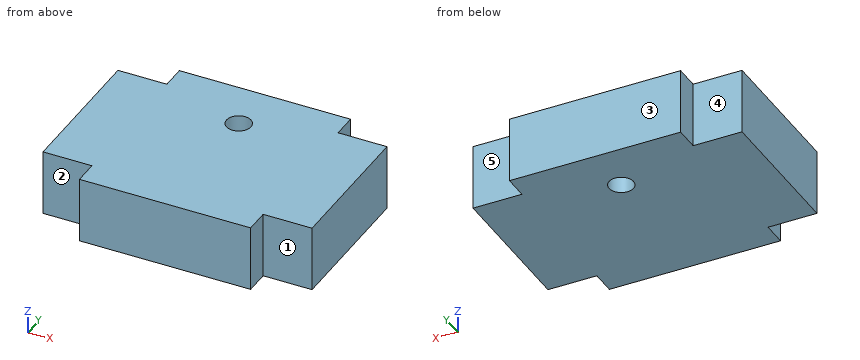
Autodesk Inventor part; units mm, degrees
ref_plane "YZ Plane" through (0, 0, 0) normal (1, 0, 0) x (0, 1, 0)
ref_plane "XZ Plane" through (0, 0, 0) normal (0, 1, 0) x (-1, 0, 0)
ref_plane "XY Plane" through (0, 0, 0) normal (0, 0, 1) x (1, 0, 0)
sketch "Sketch1" plane through (0, 0, 0) normal (0, 0, 1) x (1, 0, 0)
  line L0 (-8.75, -10) -> (8.75, -10)
  line L1 (8.75, -10) -> (8.75, 10)
  line L2 (8.75, 10) -> (-8.75, 10)
  line L3 (-8.75, 10) -> (-8.75, -10)
  line L4 (8.75, 7.5) -> (13.75, 7.5)
  line L5 (13.75, 7.5) -> (13.75, -7.5)
  line L6 (13.75, -7.5) -> (8.75, -7.5)
  line L7 (8.75, -7.5) -> (8.75, 7.5)
  line L8 (-8.75, 7.5) -> (-13.75, 7.5)
  line L9 (-13.75, 7.5) -> (-13.75, -7.5)
  line L10 (-13.75, -7.5) -> (-8.75, -7.5)
  line L11 (-8.75, -7.5) -> (-8.75, 7.5)
  circle A0 centre (0, 4.75) radius 1.25
  point P0 (0, 0)
  point P1 (8.75, 0)
  point P2 (0, 10)
  point P3 (-13.75, 0)
  point P4 (13.75, 0)
  dimension "d0" = 5
  dimension "d1" = 17.5
  dimension "d2" = 20
  dimension "d3" = 15
  dimension "d7" = 8.75
  dimension "d9" = 2.5
  dimension "d10" = 2.5
  dimension "d11" = 4.75
extrude "Extrusion1" add sketch "Sketch1" along normal blind 6.731
equation "\"d7\" = 0.5 * d1"
equation "\"d4\" = THICKB"
equation "\"THICKA\" = 3.175"
equation "\"THICKB\" = 6.731"
equation "\"THICKC\" = 12.7"
equation "\"BALLDIA\" = 12"
equation "\"MAGDIA\" = 9.5"
properties part number "Air2D_Front_Feed"
Part model, mm, in its own coordinate system. Face numbers are marked on the shaded views. A direction names the side the tool comes from. Give positions to 0.01 mm unless a question says otherwise; leave off trailing zeros. Order: outer loops, then holes, each group sorted by start corner. A loop starts at its lowest first (then second) coordinate and runs counter-clockwise, first axis right, second up. Notation, with made-up numbers: (4.25, -19) - (15.25, -19) arc R16 cw to (15.25, -7) - close; hole circle Ø1 at (-16.75, 20.5). An arc over 180 degrees is marked (long way). One line per question, with ' | ' between items.
1. Band-saw the part on B-B on x = 0. List the corners of the cut face in (y, z), then the cut area to 3 significant figures.
Filled in:
outline: (-10, 0) - (3.5, 0) - (3.5, 6.73) - (-10, 6.73) - close; (6, 0) - (10, 0) - (10, 6.73) - (6, 6.73) - close | area: 118 mm²
2. Band-saw the part on A-A on z = 4.25. List the corners of the cut face in (x, y), then the cut area to 3 significant figures.
Filled in:
outline: (-13.75, -7.5) - (-8.75, -7.5) - (-8.75, -10) - (8.75, -10) - (8.75, -7.5) - (13.75, -7.5) - (13.75, 7.5) - (8.75, 7.5) - (8.75, 10) - (-8.75, 10) - (-8.75, 7.5) - (-13.75, 7.5) - close; hole circle Ø2.5 at (0, 4.75) | area: 495 mm²
3. Drop flat-ended pins along their axis: P1, Ø3, axis at y = -9.5, z = 4.5, coming from the -X side; P2, Ø2, axis at y = -9, z = 3.5, coming from the +X side; P3, Ø4, axis at x = 12, z = 3, coming from the -Y side; P4, Ø2, axis at x = 0, y = 4.75, coming from the +Z side. Give the stop position or say it passes through.
Filled in:
P1: x = -8.75 | P2: x = 8.75 | P3: y = -7.5 | P4: through
4. Band-saw the part on C-C on y = 4.75. List the corners of the cut face in (x, z), then the cut area to 3 significant figures.
Filled in:
outline: (-13.75, 0) - (-1.25, 0) - (-1.25, 6.73) - (-13.75, 6.73) - close; (1.25, 0) - (13.75, 0) - (13.75, 6.73) - (1.25, 6.73) - close | area: 168 mm²
5. Drill centre lines: probe 1 along Y at (x, z) = (0, 2.5); probe 2 along Y at (x, z) = (11, 6.5); probe 3 along X at (y, z) = (9, 1.25). Where is each one in solid material? Low to high.
Filled in:
probe 1: -10 to 3.5, 6 to 10 | probe 2: -7.5 to 7.5 | probe 3: -8.75 to 8.75
6. Band-saw the part on D-D on y = 8.5. List the corners of the cut face in (x, z), then the cut area to 3 significant figures.
Filled in:
outline: (-8.75, 0) - (8.75, 0) - (8.75, 6.73) - (-8.75, 6.73) - close | area: 118 mm²
7. Which spindle directions (+Z, -Z, +X, -X, +Y, -Y) get a long thin tool onto all of the face, cutting with end or side? Do the marked faces 1, 2, 3, 4 and 5. Say none if no direction does.
Filled in:
face 1: +Z, -Z, +X, -Y | face 2: +Z, -Z, -X, -Y | face 3: +Z, -Z, +X, -X, +Y | face 4: +Z, -Z, -X, +Y | face 5: +Z, -Z, +X, +Y
